Geometry: final body of the model. Coordinates: model frame, mm. Face numbers are marked on the shaded views. A direction names the side the tool comes from. Give positions to 0.01 mm unless a question says otherwise; leave off trailing zeros. Loops run counter-clockwise (first coordinate to the right, second up) from the corner with the lowest first, then second, coordinate; pieces in that order, holes last. Notation, with made-up numbers: (82.25, -27.5) - (140.25, -27.5) arc R14 cw to (140.25, -3.5) - close; hole circle Ø8 at (31.5, 0). An arc over 180 degrees is marked (long way). Answer in a Markdown table with one row per item.
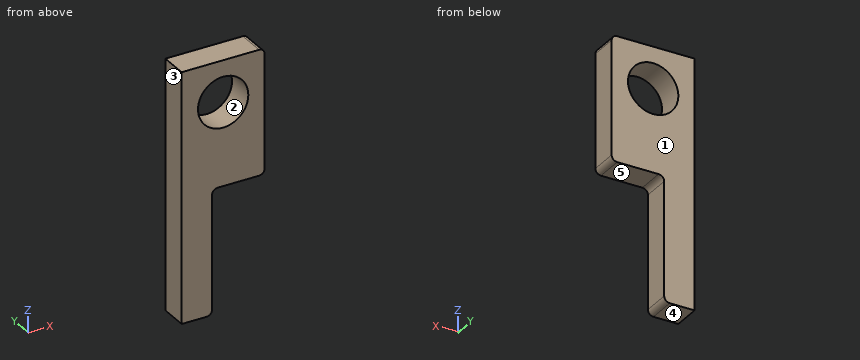
from build123d import *

# Parameters (mm, degrees)
F1_DEPTH = 10
F2_R     = 2
F3_R     = 9.1
F4_DEPTH = 25


with BuildPart() as f1:
    # F0 (on Front) → F1 (new body)
    with BuildSketch(Plane.XZ):
        Polygon((0, -45), (0, 0), (-30, 0), (-30, -90), (-19, -90), (-19, -45), align=None)
    extrude(amount=F1_DEPTH)

    # F2
    f2_edges = [f1.edges().sort_by_distance(p)[0] for p in [
        (-19, -5, -90),
        (0, -5, -45),
        (-19, -5, -45),
        (0, -5, 0),
    ]]
    fillet(f2_edges, radius=F2_R)

    # F3 (on face) → F4 (cut)
    with BuildSketch(Plane.XZ.offset(10)):
        with Locations((-15, -15)):
            Circle(F3_R)
    extrude(amount=-F4_DEPTH, mode=Mode.SUBTRACT)


solid = f1.part
Q1. Cut plane A-A (x = -15). Output: boundary loops of the cut face in (y, z).
Check values:
| item | result |
|---|---|
| outline | (-10, -45) - (0, -45) - (0, -24.1) - (-10, -24.1) - close; (-10, -5.9) - (0, -5.9) - (0, 0) - (-10, 0) - close |
Q2. Material intervals for line 1 along Z through (x, y) = (-15, -4); line 2 along X through (y, z) = (-4.5, -19.5); line 3 along Z through (x, y) = (-20.5, -9.5), sorted ascending.
Check values:
| item | result |
|---|---|
| line 1 | -45 to -24.1, -5.9 to 0 |
| line 2 | -30 to -22.91, -7.09 to 0 |
| line 3 | -89.94 to -22.25, -7.75 to 0 |
Q3. Cut plane B-B (z = -15). Output: boundary loops of the cut face in (x, y).
Check values:
| item | result |
|---|---|
| outline | (-30, -10) - (-24.1, -10) - (-24.1, 0) - (-30, 0) - close; (-5.9, -10) - (0, -10) - (0, 0) - (-5.9, 0) - close |
Q4. Draft query along X for the marked faces 1, 2 and 3. Return one class per face: pulls with the +X half, pulls with the -X half, needs draft (parallel to the pull), parting line crosses it, or undercut.
Check values:
| item | result |
|---|---|
| face 1 | needs draft |
| face 2 | undercut |
| face 3 | pulls with the -X half |
Q5. First-contact query: pin 1 (3 mm diameter, centred on y = -5.5, z = -67, fed in from +X); pin 2 (3 mm diameter, centred on x = -9, y = -5, fed in from -Z). Flat tips, straight axial feed; report the tip coordinate or a pass-through.
Check values:
| item | result |
|---|---|
| pin 1 | x = -19 |
| pin 2 | z = -45 |
Q6. Cut plane C-C (y = -2.25). Output: boundary loops of the cut face in (x, z), and give its area (3 significant figures).
Check values:
| item | result |
|---|---|
| outline | (-30, -90) - (-21, -90) arc R2 ccw to (-19, -88) - (-19, -47) arc R2 cw to (-17, -45) - (-2, -45) arc R2 ccw to (0, -43) - (0, -2) arc R2 ccw to (-2, 0) - (-30, 0) - close; hole circle Ø18.2 at (-15, -15) |
| area | 1,580 mm² |
Q7. Cut plane D-D (z = -56.5). Output: boundary loops of the cut face in (x, y), and give its area (3 significant figures).
Check values:
| item | result |
|---|---|
| outline | (-30, -10) - (-19, -10) - (-19, 0) - (-30, 0) - close |
| area | 110 mm² |
Q8. Reachability of the marked faces 4 and 5 from +Z, -Z, +X, -X, +Y, -Y: full face, straight path, thin tool, end or side. Return the list, or none.
Check values:
| item | result |
|---|---|
| face 4 | -Z, +X, -X, +Y, -Y |
| face 5 | -Z, +X, +Y, -Y |
